```python
from build123d import *

# Parameters (mm, degrees)
F0_W     = 250
F0_H     = 250
F1_DEPTH = 20
F2_W     = 10
F2_H     = 20
F2_W_2   = 250
F2_W_3   = 9.5461905003
F3_DEPTH = 150
F4_W     = 105
F4_H     = 50
F4_W_2   = 250
F5_DEPTH = 20
F7_R     = 300
F8_DEPTH = 20


with BuildPart() as f1:
    # F0 (on Top) → F1 (new body)
    with BuildSketch(Plane.XY):
        Rectangle(F0_W, F0_H)
    extrude(amount=F1_DEPTH)

    # F2 (on face) → F3 (join, symmetric)
    with BuildSketch(Plane.XY.offset(20)):
        Polygon((-145, -125), (-125, -125), (-125, 125), (-135, 125), (-135, 145), (-145, 145), align=None)
        with Locations((-130, 135)):
            Rectangle(F2_W, F2_H)
        with Locations((0, 135)):
            Rectangle(F2_W_2, F2_H)
        with Locations((129.7730952501, 135)):
            Rectangle(F2_W_3, F2_H)
        Polygon((125, 125), (125, -125), (145, -125), (145, 145), (134.5461905003, 145), (134.5461905003, 125), align=None)
    extrude(amount=F3_DEPTH, both=True)

    # F4 (on face) → F5 (join)
    with BuildSketch(Plane.XY.offset(170)):
        with Locations((-197.5, 89.5141008463)):
            Rectangle(F4_W, F4_H)
        with Locations((-197.5, -18.0167201906)):
            Rectangle(F4_W, F4_H)
        with Locations((0, -18.0167201906)):
            Rectangle(F4_W_2, F4_H)
        with Locations((0, 89.5141008463)):
            Rectangle(F4_W_2, F4_H)
        with Locations((197.5, 89.5141008463)):
            Rectangle(F4_W, F4_H)
        with Locations((197.5, -18.0167201906)):
            Rectangle(F4_W, F4_H)
    extrude(amount=-F5_DEPTH)

    # F7 (on offset) → F8 (join)
    with BuildSketch(Plane.XY.offset(190)):
        with Locations((0, -10.6063758958)):
            Circle(F7_R)
    extrude(amount=-F8_DEPTH)


solid = f1.part
```
Input: part model. Units: mm. Frame: model coordinates. A direction names the side the tool comes from. Give positions to 0.01 mm unless a question says otherwise; leave off trailing zeros. Order: outer loops, then holes, each group sorted by start corner. A loop starts at its lowest first (then second) coordinate and runs counter-clockwise, first axis right, second up. Notation, with made-up numbers: M -30.5,-13.5 L 5.5,-13.5 A35 cw 5.5,20.5 Z; hole C 51.25,28 d7. An arc over 180 degrees is marked long. Return JSON: item names as keys, results as strings.
Item 1: Cut plane B-B (x = 0). Return loops of the section in (y, z).
Solutions:
{"outline": "M -310.61,170 L -43.02,170 L -43.02,150 L 6.98,150 L 6.98,170 L 64.51,170 L 64.51,150 L 114.51,150 L 114.51,170 L 125,170 L 125,20 L -125,20 L -125,0 L 125,0 L 125,-130 L 145,-130 L 145,170 L 289.39,170 L 289.39,190 L -310.61,190 Z"}
Item 2: First-contact query: P1, Ø6, axis at x = 68, z = 34, coming from the +Y side; P2, Ø8, axis at x = 176, y = 217, coming from the -Z side; P3, Ø6, axis at x = -216, z = 162.5, coming from the -Y side. Flat tips, straight axial feed; report the tip coordinate or a pass-through.
Solutions:
{"P1": "y = 145", "P2": "z = 170", "P3": "y = -43.02"}
Item 3: Pull-direction query (Z, two-part tool) for faces 4 (the flat face through (-2, 125, 96)), 5 (the flat face through (-198, 64.514, 160)), 6 (the flat face through (-198, 90, 150)); classes: +Z half, -Z half, draft (parallel to the pull), parting line (faces both ways), or undercut.
Solutions:
{"face 4": "undercut", "face 5": "draft", "face 6": "-Z half"}
Item 4: Access query for faces 1 (the flat face through (-198, 114.514, 160)), 2 (the flat face through (-250, -18, 160)), 3 (the flat face through (-2, -43.017, 160)). Directions: +Z, -Z, +X, -X, +Y, -Y. A direction counts if a zero-diameter tool reaches every point of the face in a straight line with its end or side. Return the directions, or none.
Solutions:
{"face 1": "-Z, -X, +Y", "face 2": "-Z, -X, +Y, -Y", "face 3": "-Y"}
Item 5: Cut plane D-D (x = -215). Return loops of the section in (y, z).
Solutions:
{"outline": "M -219.83,170 L -43.02,170 L -43.02,150 L 6.98,150 L 6.98,170 L 64.51,170 L 64.51,150 L 114.51,150 L 114.51,170 L 198.62,170 L 198.62,190 L -219.83,190 Z"}
Item 6: Cut plane C-C (y = 54). Return loops of the section in (x, z), then the cut area to 3 significant figures.
Solutions:
{"outline": "M -292.96,170 L -145,170 L -145,-130 L -125,-130 L -125,0 L 125,0 L 125,-130 L 145,-130 L 145,170 L 292.96,170 L 292.96,190 L -292.96,190 Z; hole M -125,20 L 125,20 L 125,170 L -125,170 Z", "area": "28,700 mm^2"}
Item 7: Ray query, probe 1 along Z at (x, y) = (13.5, 78); probe 2 along Z at (x, y) = (-50.5, -138); probe 3 along X at (y, z) = (-124, 36). Return the intervals inside material, ascending.
Solutions:
{"probe 1": "0 to 20, 150 to 190", "probe 2": "170 to 190", "probe 3": "-145 to -125, 125 to 145"}
Item 8: Cut plane A-A (z = -71.5). Return loops of the section in (x, y).
Solutions:
{"outline": "M -145,-125 L -125,-125 L -125,125 L 125,125 L 125,-125 L 145,-125 L 145,145 L -145,145 Z"}
